Source: three-view drawing plus pictorial views. Frame: mm from the lowest corner of the part. Give positions to 0.01 mm unless a question says otherwise; leave off trailing zeros. Order: outer loops, then holes, each group sorted by start corner. A loop starts at its lowest first (then second) coordinate and runs counter-clockwise, first axis right, second up. Notation, with made-up numbers: (26.5, 61.25) - (82.5, 61.25) arc R24 cw to (82.5, 72.25) - close; hole circle Ø4 at (52.5, -8). An arc over 180 degrees is marked (long way). Use one line per item in the form item = value.
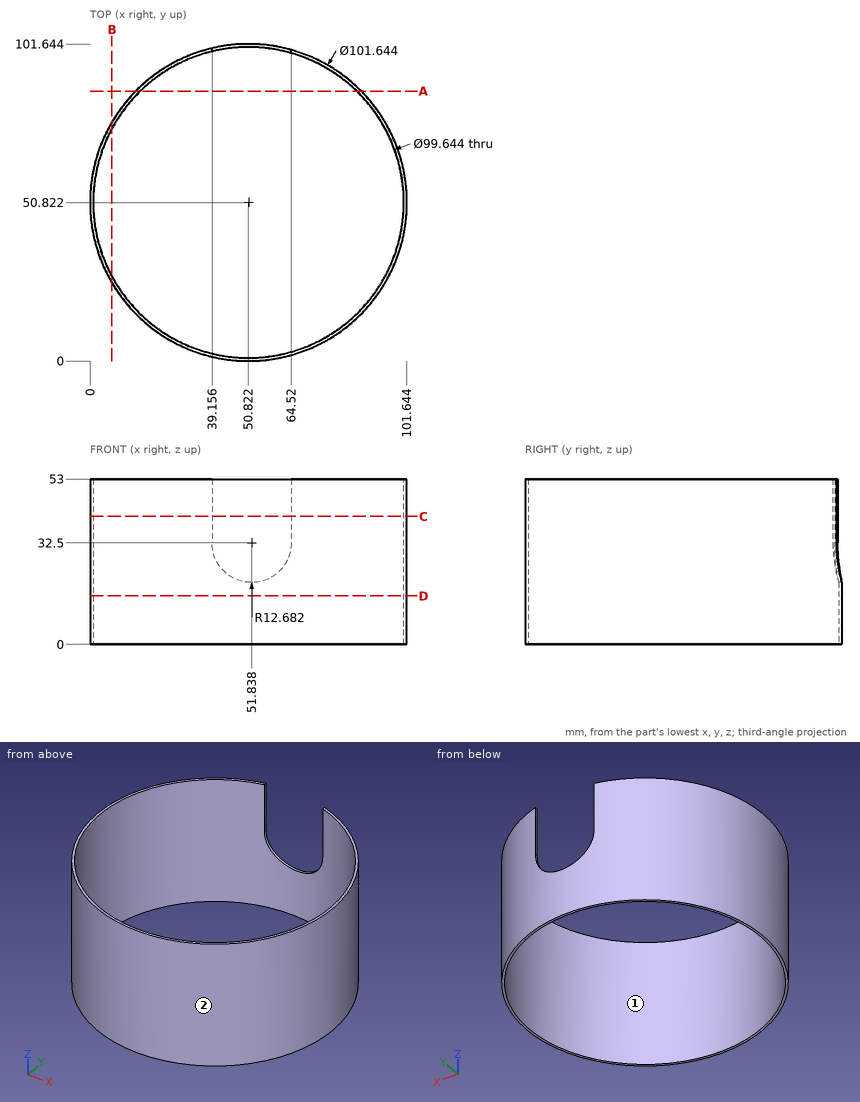
(1) Ray query, line 1 along Y through (x, z) = (23, 47.5); line 2 along X through (y, z) = (70, 48) (3 decimals); line 3 along X through (y, z) = (71, 38.5). Return the intervals inside material, ascending.
Computed values:
line_1 = 8.29 to 9.49, 92.15 to 93.35
line_2 = 3.757 to 4.839, 96.805 to 97.887
line_3 = 4.18 to 5.27, 96.38 to 97.47
(2) Cut plane A-A on y = 86.5. Output: boundary loops of the cut face in (x, z).
Computed values:
outline = (14.63, 0) - (16.05, 0) - (16.05, 53) - (14.63, 53) - close; (85.6, 0) - (87.02, 0) - (87.02, 53) - (85.6, 53) - close
(3) Cut plane B-B on x = 7. Output: boundary loops of the cut face in (y, z), plus the area to 3 significant figures.
Computed values:
outline = (25.08, 0) - (27.12, 0) - (27.12, 53) - (25.08, 53) - close; (74.53, 0) - (76.56, 0) - (76.56, 53) - (74.53, 53) - close
area = 216 mm²
(4) Pull-direction query (X, two-part tool) for the marked faces 1 and 2; classes: released by +X, released by -X, zero draft, split by the parting line, or undercut.
Computed values:
face_1 = undercut
face_2 = split by the parting line
(5) Cut plane D-D on z = 15.5. Output: boundary loops of the cut face in (x, y), plus the area to 3 significant figures.
Computed values:
outline = circle Ø101.64 at (50.82, 50.82); hole circle Ø99.64 at (50.82, 50.82)
area = 316 mm²
(6) Cut plane C-C on z = 41. Output: boundary loops of the cut face in (x, y).
Computed values:
outline = (39.16, 99.26) - (39.16, 100.29) arc R50.82 ccw (long way) to (64.52, 99.76) - (64.52, 98.72) arc R49.82 cw (long way) to start
(7) Contact query for flat-ended pins moving along their axis: pin 1 Ø6 at (y, z) = (67, 44) entering from +X; pin 2 Ø2 at (x, z) = (74, 9.5) entering from +Y; pin 3 Ø1.5 at (x, z) = (47, 21.5) entering from +Y. Output: stop coordinate, or through.
Computed values:
pin_1 = 99.91
pin_2 = 96.55
pin_3 = 101.5
